The drawing under review shows one solid part. Ordinate dimensions are in mm from its lowest x, y, z. A direction names the side the tool comes from. Coordinates: 2 decimals unless noted, no trailing zeros. Write each loop counter-clockwise with the first axis right and the second up, starting at its lowest first coordinate (ties: lowest second). Pieces come first, ordered by that corner, then holes.
Q1. Take a section at A-A (z = 9.5). Give the boundary of the cut face in (x, y) (1 decimal).
Q2. Machinability: for the marked faces 1 and 2, which of the approach directions +Z, -Z, +X, -X, +Y, -Y give a long, thin tool a straight path to every point of the face, cutting with its end or side? Answer none if there is none.
Q3. Take a section at D-D (x = 42). Give the boundary of the cut face in (y, z).
Q4. For probe 1 along Y at (x, z) = (28.5, 13) (1 decimal); probe 2 along X at (y, z) = (45, 6); probe 3 along Y at (x, z) = (28, 2) (1 decimal), list the stretches that pass through material, from the lowest coordinate up.
Q5. Take a section at C-C (y = 39). Give the boundary of the cut face in (x, z).
Q6. Mouldability with a two-part tool opening along X and no side actions: class the marked faces 3, 4, 5 and 6 as pulls with the +X half, pulls with the -X half, needs draft (parallel to the pull), parting line crosses it, or undercut.
Q7. Take a section at B-B (x = 25). Give the boundary of the cut face in (y, z), and give its area (3 significant figures).
Q8. Insertion check: pin 1 (6 mm diameter, centred on x = 29.5, z = 10, fed in from -Y); pin 2 (3 mm diameter, centred on y = 22.5, z = 10.5, fed in from -X). Each pin has a flat end and moves straight along its axis. Give the tip position at first contact, or say it passes through.
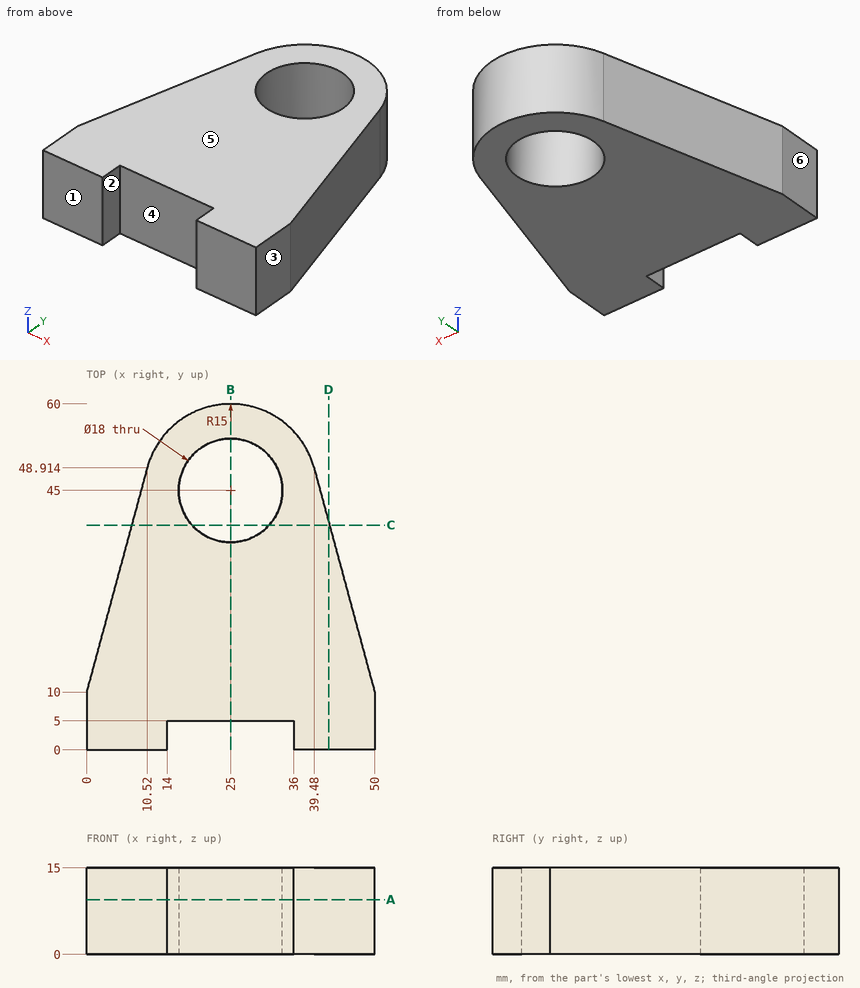
Response:
1. outline: (0, 0) - (14, 0) - (14, 5) - (36, 5) - (36, 0) - (50, 0) - (50, 10) - (39.5, 48.9) arc R15 ccw to (10.5, 48.9) - (0, 10) - close; hole circle Ø18 at (25, 45)
2. face 1: +Z, -Z, +X, -X, -Y
2. face 2: +Z, -Z, -Y
3. outline: (0, 0) - (39.59, 0) - (39.59, 15) - (0, 15) - close
4. probe 1: y = 5 to 36.7, 53.3 to 59.6
4. probe 2: x = 9.46 to 16, 34 to 40.54
4. probe 3: y = 5 to 36.5, 53.5 to 59.7
5. outline: (7.84, 0) - (18.29, 0) - (18.29, 15) - (7.84, 15) - close; (31.71, 0) - (42.16, 0) - (42.16, 15) - (31.71, 15) - close
6. face 3: pulls with the +X half
6. face 4: undercut
6. face 5: needs draft
6. face 6: pulls with the -X half
7. outline: (5, 0) - (36, 0) - (36, 15) - (5, 15) - close; (54, 0) - (60, 0) - (60, 15) - (54, 15) - close
7. area: 555 mm2
8. pin 1: stops at y = 5
8. pin 2: stops at x = 2.97
